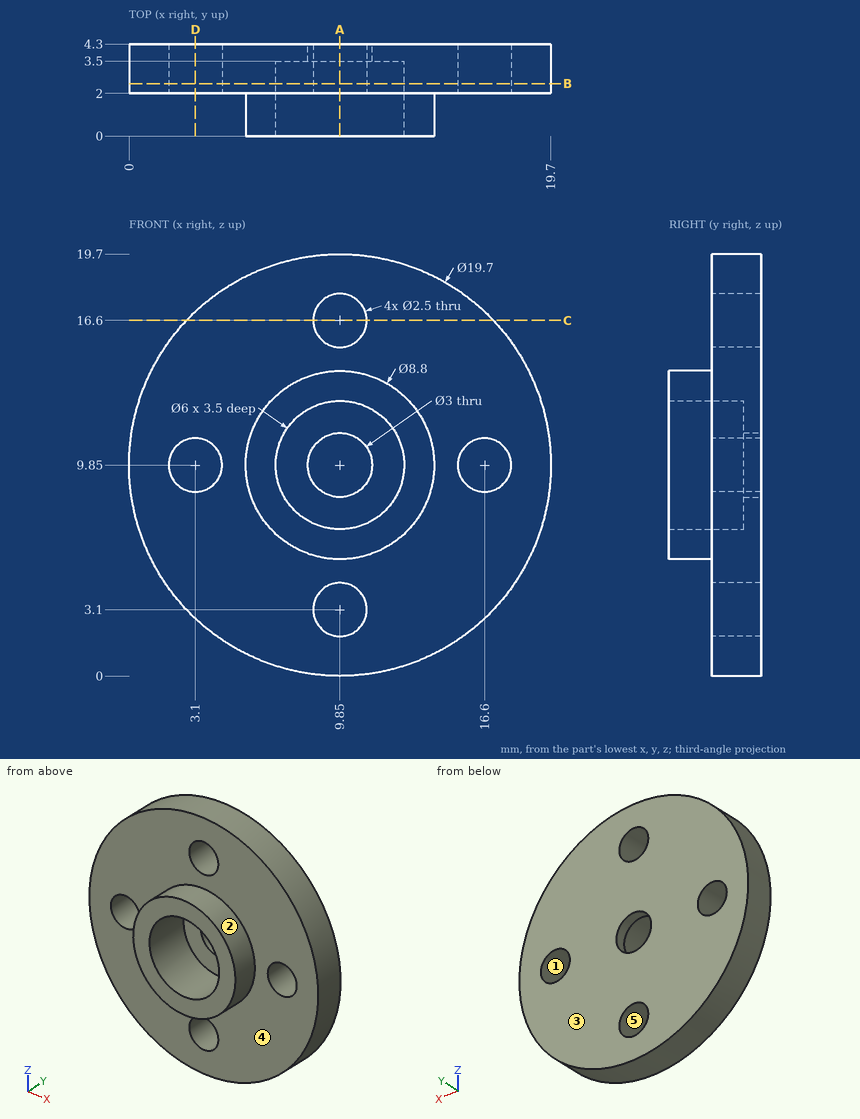
Could you check a few things on this drawing? It's one solid part, dimensions in mm from its lowest x, y, z. A direction names the side the tool comes from. Round coordinates to 2 decimals unless told otherwise and drop trailing zeros. Write each loop counter-clockwise with the first axis right and the second up, starting at its lowest first coordinate (ties: lowest second). Pieces come first, ordered by that corner, then holes. Notation, with made-up numbers: (16.25, 7) -> (71.25, 7) arc R5 ccw to (71.25, 11) -> close; hole circle Ø1 at (57.5, 17). An arc over 180 degrees is marked (long way). Use one line per item in the form item = value. Start each with the question number.
Q1. Which directions (+Z, -Z, +X, -X, +Y, -Y) give clear straight access to the entire face, cutting with the end or side of a thin tool? Please do the marked faces 4 and 5.
Q2. We'd pull the mould along X, two halves only. Please class the marked faces 1, 2 and 3: +X half, -X half, draft (parallel to the pull), parting line (faces both ways), or undercut.
Q3. Imagine slicing it at C-C (z = 16.6). Please give me the cut outline in (x, y), then the cut area to 3 significant figures.
Q4. Imagine slicing it at D-D (x = 3.1). Please give me the cut outline in (y, z).
Q5. I'm going to push flat-ended pins straight in: P1, Ø2, axis at x = 13.5, y = 3.5, coming from the -Z side; P2, Ø5, axis at x = 9.85, z = 9.85, coming from the -Y side; P3, Ø6.5, axis at x = 10, z = 10, coming from the -Y side. Where does each tip first touch, or does it pass through?
Q6. If I drill on probe 1 along X at (y, z) = (3.8, 9.85); probe 2 along Y at (x, z) = (14, 2.25); probe 3 along Z at (x, y) = (9.25, 4.1), over which ranges is the centre line in solid material (lowest first)? Write a range as [from, to].
Q7. Imagine slicing it at B-B (y = 2.45). Please give me the cut outline in (x, z).
Q8. Imagine slicing it at A-A (x = 9.85). Please give me the cut outline in (y, z), then the cut area to 3 significant figures.
Worked out:
q1.face_4 = -Y
q1.face_5 = +Y, -Y
q2.face_1 = undercut
q2.face_2 = parting line
q2.face_3 = draft
q3.outline = (2.68, 2) -> (8.6, 2) -> (8.6, 4.3) -> (2.68, 4.3) -> close; (11.1, 2) -> (17.02, 2) -> (17.02, 4.3) -> (11.1, 4.3) -> close
q3.area = 27.2 mm^2
q4.outline = (2, 2.68) -> (4.3, 2.68) -> (4.3, 8.6) -> (2, 8.6) -> close; (2, 11.1) -> (4.3, 11.1) -> (4.3, 17.02) -> (2, 17.02) -> close
q5.P1 = 0.36
q5.P2 = 3.5
q5.P3 = 0
q6.probe_1 = [0, 1.85], [4.35, 8.35], [11.35, 15.35], [17.85, 19.7]
q6.probe_2 = [2, 4.3]
q6.probe_3 = [0.02, 2], [4.2, 8.48], [11.22, 15.5], [17.7, 19.68]
q7.outline = circle Ø19.7 at (9.85, 9.85); hole circle Ø2.5 at (3.1, 9.85); hole circle Ø6 at (9.85, 9.85); hole circle Ø2.5 at (9.85, 3.1); hole circle Ø2.5 at (9.85, 16.6); hole circle Ø2.5 at (16.6, 9.85)
q8.outline = (0, 5.45) -> (2, 5.45) -> (2, 4.35) -> (4.3, 4.35) -> (4.3, 8.35) -> (3.5, 8.35) -> (3.5, 6.85) -> (0, 6.85) -> close; (0, 12.85) -> (3.5, 12.85) -> (3.5, 11.35) -> (4.3, 11.35) -> (4.3, 15.35) -> (2, 15.35) -> (2, 14.25) -> (0, 14.25) -> close; (2, 0) -> (4.3, 0) -> (4.3, 1.85) -> (2, 1.85) -> close; (2, 17.85) -> (4.3, 17.85) -> (4.3, 19.7) -> (2, 19.7) -> close
q8.area = 28.0 mm^2
